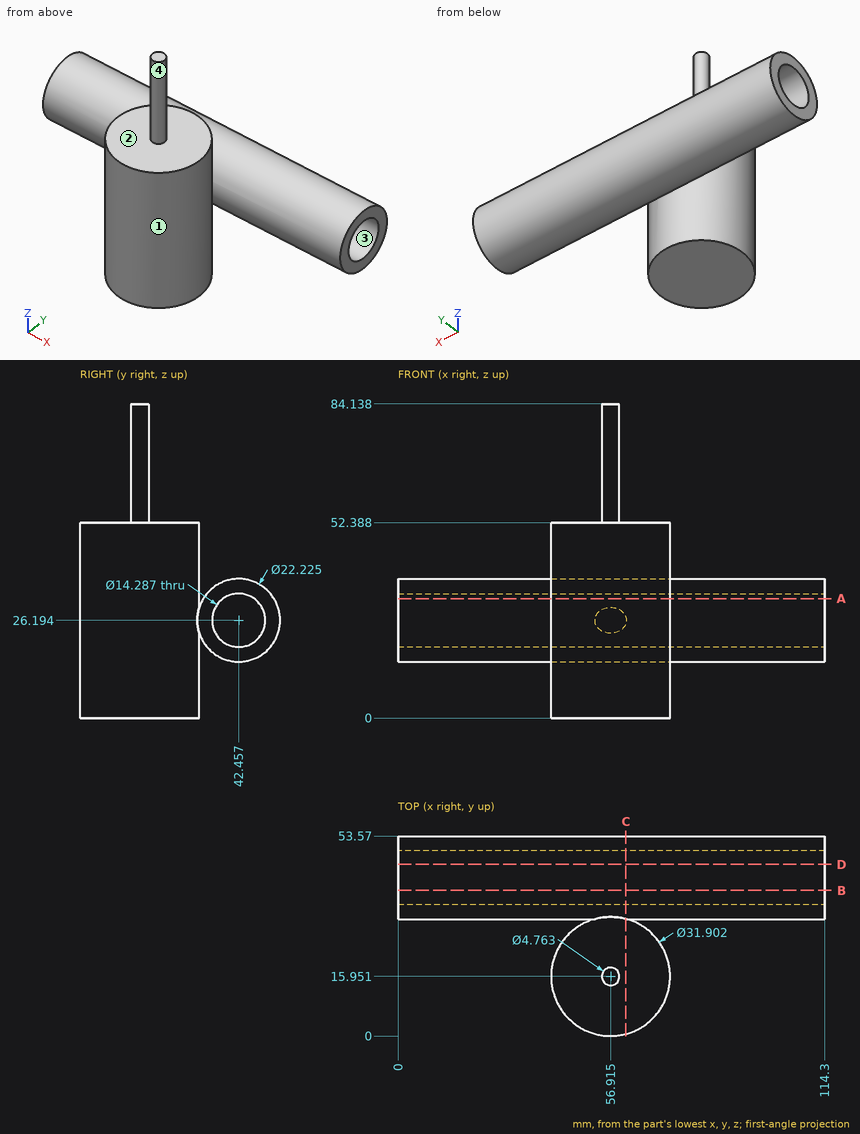
Geometry check sheet. Reference: drawing and pictorial views, mm from the part's lowest x, y, z. Round coordinates to 2 decimals unless told otherwise and drop trailing zeros. Loops run counter-clockwise (first coordinate to the right, second up) from the corner with the lowest first, then second, coordinate; pieces in that order, holes last. Notation, with made-up numbers: (9, -38.75) - (28, -38.75) arc R26 cw to (28, -12.75) - close; hole circle Ø9 at (87.5, -5). An arc over 180 degrees is marked (long way). Use a Markdown table: item, result. Add a question column.
1. Gauge pin test, flat ends, axial feed: pin 1 (5 mm diameter, centred on y = 32, z = 11, fed in from +X) (1 decimal); pin 2 (1 mm diameter, centred on y = 14.5, z = 63.5, fed in from -X); pin 3 (11.5 mm diameter, centred on y = 42.46, z = 26.19, fed in from -X); pin 4 (1 mm diameter, centred on x = 38.5, y = 42, fed in from +Z). Record the tip position at first contact, or that the pin passes through.
2. Section check A-A, the plane z = 32. Give the number of separate pieces and of enclosed holes in the cut face, plus the area to 3 significant figures.
3. Section check C-C, the plane x = 61. Record the boundary of the cut face in (y, z) (1 decimal), plus the area to 3 significant figures.
4. Thickness scan on probe 1 along Z at (x, y) = (89.5, 42) (1 decimal); probe 2 along Z at (x, y) = (52.5, 5); probe 3 along Z at (x, y) = (108, 45.5) (1 decimal). Record the ranges inside material, lowest first. Write a range as [from, to].
5. Section check D-D, the plane y = 46. Record the boundary of the cut face in (x, z).
6. Section check B-B, the plane y = 39. Record the boundary of the cut face in (x, z) (1 decimal).
7. Release check for a two-part mould opening along Y. For the marked faces 1, 2, 3 and 4 record: released by +Y, released by -Y, zero draft, split by the parting line, or undercut.
Checks:
| question | item | result |
|---|---|---|
| 1 | pin 1 | stops at x = 65.3 |
| 1 | pin 2 | stops at x = 54.73 |
| 1 | pin 3 | passes through |
| 1 | pin 4 | stops at z = 37.31 |
| 2 | separate pieces | 3 |
| 2 | enclosed holes | 0 |
| 2 | area | 2,010 mm^2 |
| 3 | outline | (0.5, 0) - (31.4, 0) - (31.4, 25.4) arc R11.1 ccw (long way) to (31.4, 26.9) - (31.4, 52.4) - (0.5, 52.4) - close; hole circle Ø14.3 at (42.5, 26.2) |
| 3 | area | 1,840 mm^2 |
| 4 | probe 1 | z = [15.1, 19.1], [33.3, 37.3] |
| 4 | probe 2 | z = [0, 52.39] |
| 4 | probe 3 | z = [15.5, 19.7], [32.7, 36.9] |
| 5 | outline | (0, 15.66) - (114.3, 15.66) - (114.3, 19.99) - (0, 19.99) - close; (0, 32.4) - (114.3, 32.4) - (114.3, 36.73) - (0, 36.73) - close |
| 6 | outline | (0, 15.6) - (114.3, 15.6) - (114.3, 19.9) - (0, 19.9) - close; (0, 32.4) - (114.3, 32.4) - (114.3, 36.8) - (0, 36.8) - close |
| 7 | face 1 | undercut |
| 7 | face 2 | zero draft |
| 7 | face 3 | undercut |
| 7 | face 4 | split by the parting line |
